from build123d import *

# Parameters (mm, degrees)
F0_W      = 203.207492
F0_H      = 228.935466
F1_DEPTH  = 152.4
F2_W      = 175.73382
F2_H      = 202.479318
F3_DEPTH  = 1270
F4_W      = 204.225034
F4_H      = 228.935466
F5_DEPTH  = 25.4
F6_R      = 74.025585
F7_DEPTH  = 101.6
F8_R      = 62.584058
F9_DEPTH  = 12700
F10_W     = 204.514414
F10_H     = 227.628558
F11_DEPTH = 25.4
F12_W     = 130.283504
F12_H     = 17.982788
F13_DEPTH = 12700
F14_W     = 153.912366
F14_H     = 17.956443
F15_DEPTH = 127000


with BuildPart() as f1:
    # F0 (on Top) → F1 (new body)
    with BuildSketch(Plane.XY):
        Rectangle(F0_W, F0_H)
    extrude(amount=F1_DEPTH)

    # F2 (on Top) → F3 (cut, symmetric)
    with BuildSketch(Plane.XY):
        Rectangle(F2_W, F2_H)
    extrude(amount=F3_DEPTH, both=True, mode=Mode.SUBTRACT)

    # F4 (on Top) → F5 (join)
    with BuildSketch(Plane.XY):
        Rectangle(F4_W, F4_H)
    extrude(amount=F5_DEPTH)

    # F6 (on Top) → F7 (join)
    with BuildSketch(Plane.XY):
        Circle(F6_R)
    extrude(amount=F7_DEPTH)

    # F8 (on Top) → F9 (cut, symmetric)
    with BuildSketch(Plane.XY):
        Circle(F8_R)
    extrude(amount=F9_DEPTH, both=True, mode=Mode.SUBTRACT)

    # F10 (on Top) → F11 (join)
    with BuildSketch(Plane.XY):
        Rectangle(F10_W, F10_H)
    extrude(amount=F11_DEPTH)

    # F12 (on Front) → F13 (cut, symmetric)
    with BuildSketch(Plane.XZ):
        with Locations((2.752468, 123.610016)):
            Rectangle(F12_W, F12_H)
    extrude(amount=F13_DEPTH, both=True, mode=Mode.SUBTRACT)

    # F14 (on Right) → F15 (cut, symmetric)
    with BuildSketch(Plane.YZ):
        with Locations((-2.931662, 131.546791)):
            Rectangle(F14_W, F14_H)
    extrude(amount=F15_DEPTH, both=True, mode=Mode.SUBTRACT)


solid = f1.part
Read the model definition and answer for the solid it produces. Units are mm, in the model's axes. A direction names the side the tool comes from. Round coordinates to 2 decimals unless told otherwise and drop trailing zeros. Write each loop counter-clockwise with the first axis right and the second up, starting at its lowest first coordinate (ties: lowest second). Pieces come first, ordered by that corner, then holes. Notation, with made-up numbers: (-7, 50.5) - (35, 50.5) arc R10 ccw to (35, 68.5) - close; hole circle Ø7 at (22.5, 23.25). An arc over 180 degrees is marked (long way). Use a Markdown table: item, result.
(1) Straight lines are drawn through the part: line 1 along Y through (x, z) = (0, 50.5); line 2 along X through (y, z) = (-87, 79); line 3 along Y through (x, z) = (-82, 144.5). For each, find the intervals that lie inside material, in ascending order. Write a range as [from, to].
Reported:
| item | result |
|---|---|
| line 1 | [-114.47, -101.24], [-74.03, -62.58], [62.58, 74.03], [101.24, 114.47] |
| line 2 | [-101.6, -87.87], [87.87, 101.6] |
| line 3 | [-114.47, -101.24], [101.24, 114.47] |
(2) The part is cut by section B-B (z = 127). Write down the section's boundary in (x, y).
Reported:
| item | result |
|---|---|
| outline | (-101.6, -114.47) - (-62.39, -114.47) - (-62.39, -101.24) - (-87.87, -101.24) - (-87.87, -79.89) - (-101.6, -79.89) - close; (-101.6, 74.02) - (-87.87, 74.02) - (-87.87, 101.24) - (-62.39, 101.24) - (-62.39, 114.47) - (-101.6, 114.47) - close; (67.89, -114.47) - (101.6, -114.47) - (101.6, -79.89) - (87.87, -79.89) - (87.87, -101.24) - (67.89, -101.24) - close; (67.89, 101.24) - (87.87, 101.24) - (87.87, 74.02) - (101.6, 74.02) - (101.6, 114.47) - (67.89, 114.47) - close |
(3) Which of the six approach directions +Z, -Z, +X, -X, +Y, -Y give full straight-line access (tool end or side, diameter ignored) to faces 3 (the flat face through (-60, 46, 25.4)), 4 (the flat face through (2, -108, 114.619)), 5 (the flat face through (102.257, -2, 13)), 6 (the flat face through (-95, 74.025, 131)), 7 (the flat face through (-91, 9, 152.4))?
Reported:
| item | result |
|---|---|
| face 3 | +Z |
| face 4 | +Y, -Y |
| face 5 | +Z, -Z, +X, +Y, -Y |
| face 6 | +X, -X |
| face 7 | +Z, +X, -X, +Y, -Y |
(4) The part is cut by section D-D (y = -93). Write down the section's boundary in (x, z).
Reported:
| item | result |
|---|---|
| outline | (-102.26, 0) - (102.26, 0) - (102.26, 25.4) - (101.6, 25.4) - (101.6, 152.4) - (87.87, 152.4) - (87.87, 25.4) - (-87.87, 25.4) - (-87.87, 152.4) - (-101.6, 152.4) - (-101.6, 25.4) - (-102.26, 25.4) - close |
(5) The mould has two halves that part along Y. Classify faces 1 (the flat face through (2, 108, 132.601)), 2 (the flat face through (-95, -4, 140.525)): released by +Y, released by -Y, zero draft, split by the parting line, or undercut.
Reported:
| item | result |
|---|---|
| face 1 | zero draft |
| face 2 | undercut |
(6) The part is cut by section C-C (y = 0). Write down the section's boundary in (x, z), then the cut area to 3 significant figures.
Reported:
| item | result |
|---|---|
| outline | (-102.26, 0) - (102.26, 0) - (102.26, 25.4) - (101.6, 25.4) - (101.6, 122.57) - (87.87, 122.57) - (87.87, 25.4) - (74.03, 25.4) - (74.03, 101.6) - (62.58, 101.6) - (62.58, 25.4) - (-62.58, 25.4) - (-62.58, 101.6) - (-74.03, 101.6) - (-74.03, 25.4) - (-87.87, 25.4) - (-87.87, 122.57) - (-101.6, 122.57) - (-101.6, 25.4) - (-102.26, 25.4) - close; (-101.6, 140.53) - (-87.87, 140.53) - (-87.87, 152.4) - (-101.6, 152.4) - close; (87.87, 140.53) - (101.6, 140.53) - (101.6, 152.4) - (87.87, 152.4) - close |
| area | 9,930 mm2 |
(7) Each of these flat-tipped pins is pushed along its axis until it touches: pin 1 Ø0.5 at (x, y) = (102, 26) entering from +Z; pin 2 Ø1.5 at (y, z) = (-17.5, 102.5) entering from -X; pin 3 Ø4 at (y, z) = (46.5, 115.5) entering from +X. Where does it stop, or does it pass through?
Reported:
| item | result |
|---|---|
| pin 1 | z = 25.4 |
| pin 2 | x = -101.6 |
| pin 3 | x = 101.6 |
(8) The part is cut by section A-A (x = 0). Write down the section's boundary in (y, z), then the cut area to 3 significant figures.
Reported:
| item | result |
|---|---|
| outline | (-114.47, 0) - (114.47, 0) - (114.47, 114.62) - (101.24, 114.62) - (101.24, 25.4) - (74.03, 25.4) - (74.03, 101.6) - (62.58, 101.6) - (62.58, 25.4) - (-62.58, 25.4) - (-62.58, 101.6) - (-74.03, 101.6) - (-74.03, 25.4) - (-101.24, 25.4) - (-101.24, 114.62) - (-114.47, 114.62) - close; (-114.47, 132.6) - (-101.24, 132.6) - (-101.24, 152.4) - (-114.47, 152.4) - close; (101.24, 132.6) - (114.47, 132.6) - (114.47, 152.4) - (101.24, 152.4) - close |
| area | 10,400 mm2 |
